Here's how the part is built. I have some questions about the finished solid (model axes, mm). A direction names the side the tool comes from. Coordinates: 2 decimals unless noted, no trailing zeros. Write each loop counter-clockwise with the first axis right and the second up, starting at its lowest first coordinate (ties: lowest second). Pieces come first, ordered by that corner, then holes.
Item 1: If we section it at B-B (x = 3.5): Please give me the cut outline in (y, z), then the cut area to 3 significant figures.
Item 2: I'm going to push flat-ended pins straight in: pin 1 Ø0.6 at (y, z) = (2, 1) entering from -X; pin 2 Ø3 at (x, y) = (30.5, 15) entering from -Z. Where does each tip first touch, or does it pass through?
Item 3: If we section it at A-A (z = 1.55): Please give me the cut outline in (x, y).
Item 4: If I drill on line 1 (Y direction, x = 27.5, z = 1.15); line 2 (Y direction, x = 2.5, z = 1.15); line 3 (Z direction, x = 7, y = 8.75), over which ranges is the centre line in solid material (lowest first)?
Item 5: For faces 1 (the face through (0, 15, 1)), 2 (the face through (5, 0.5, 1)), 3 (the face through (2, 26.35, 1)), which set-ups out of +Z, -Z, +X, -X, +Y, -Y let a thin tool reach every point of the face, with its end or its side?
Item 6: We'd pull the mould along Y, two halves only. Please class faces 4 (the face through (1, 3.15, 1)), 5 (the face through (36, 15, 2.25)), 6 (the face through (18, 0, 1)), 7 (the face through (19, 29.5, 1)): +Y half, -Y half, draft (parallel to the pull), parting line (faces both ways), or undercut.
from build123d import *

# Parameters (mm, degrees)
EXTRUDE_938_DEPTH  = 2.25
EXTRUDE_987_DEPTH  = 0.1
SKETCH_1488_W      = 28.5
SKETCH_1488_H      = 28.5
EXTRUDE_2115_DEPTH = 2.15
SKETCH_2253_W      = 1.5
SKETCH_2253_H      = 0.4
EXTRUDE_2914_DEPTH = 0.01


with BuildPart() as part:
    # Sketch 282 → Extrude 938 (new body)
    with BuildSketch(Plane.XY):
        Polygon((36.5, 29.5), (0, 29.5), (0, 26.6), (2.75, 26.6), (2.75, 29.25), (35.6, 29.25), (35.6, 0.25), (2.75, 0.25), (2.75, 2.9), (0, 2.9), (0, 0), (36.5, 0), align=None)
    extrude(amount=EXTRUDE_938_DEPTH)

    # 底面草图<3> → Extrude 987 (add)
    with BuildSketch(Plane.XY):
        Polygon((2.75, 26.6), (0, 26.6), (0, 2.9), (2.75, 2.9), (2.75, 0.25), (35.6, 0.25), (35.6, 29.25), (2.75, 29.25), align=None)
    extrude(amount=EXTRUDE_987_DEPTH)

    # Sketch 1488 → Extrude 2115 (add)
    with BuildSketch(Plane.XY.offset(0.1)):
        with Locations((21.1, 14.75)):
            Rectangle(SKETCH_1488_W, SKETCH_1488_H)
        Polygon((6.75, 0.5), (6.75, 29), (3, 29), (3, 26.35), (0, 26.35), (0, 3.15), (3, 3.15), (3, 0.5), align=None)
    extrude(amount=EXTRUDE_2115_DEPTH)

    # Sketch 2253 → Extrude 2914 (add)
    with BuildSketch(Plane(origin=(0, 0, 0), x_dir=(-1, 0, 0), z_dir=(0, 0, -1))):
        with Locations((-8.05, 9.55)):
            Rectangle(SKETCH_2253_W, SKETCH_2253_H)
        with Locations((-8.05, 19.95)):
            Rectangle(SKETCH_2253_W, SKETCH_2253_H)
    extrude(amount=EXTRUDE_2914_DEPTH)


solid = part.part
Answer list:
1. outline: (0, 0) - (29.5, 0) - (29.5, 2.25) - (29.25, 2.25) - (29.25, 0.1) - (29, 0.1) - (29, 2.25) - (0.5, 2.25) - (0.5, 0.1) - (0.25, 0.1) - (0.25, 2.25) - (0, 2.25) - close
1. area: 65.3 mm2
2. pin 1: stops at x = 0
2. pin 2: stops at z = 0
3. outline: (0, 0) - (36.5, 0) - (36.5, 29.5) - (0, 29.5) - (0, 26.6) - (2.75, 26.6) - (2.75, 29.25) - (35.6, 29.25) - (35.6, 0.25) - (2.75, 0.25) - (2.75, 2.9) - (0, 2.9) - close; (0, 3.15) - (3, 3.15) - (3, 0.5) - (6.75, 0.5) - (6.75, 29) - (3, 29) - (3, 26.35) - (0, 26.35) - close; (6.85, 0.5) - (35.35, 0.5) - (35.35, 29) - (6.85, 29) - close
4. line 1: y = 0 to 0.25, 0.5 to 29, 29.25 to 29.5
4. line 2: y = 0 to 2.9, 3.15 to 26.35, 26.6 to 29.5
4. line 3: z = 0 to 2.25
5. face 1: +Z, -Z, -X, +Y, -Y
5. face 2: +Z
5. face 3: +Z, -X
6. face 4: undercut
6. face 5: draft
6. face 6: -Y half
6. face 7: +Y half
